For this review, take the finished solid that the model builds, in its own axes (mm). Round coordinates to 2 decimals unless told otherwise and drop trailing zeros. Write each loop counter-clockwise with the first axis right and the second up, starting at its lowest first coordinate (ties: lowest second). Pieces come first, ordered by that corner, then holes. Notation, with made-up numbers: (70.25, 32) - (97.25, 32) arc R21 ccw to (97.25, 66) - close; hole circle Ø4 at (12, 42.5). An arc over 180 degrees is marked (long way). One line per item, written item: value. Start each with the question number.
Q1. Clearance check with flat-ended pins moving along their axes: pin 1 Ø3.5 at (x, y) = (-23.5, -23.5) entering from -Z; pin 2 Ø3.5 at (x, y) = (23.5, 23.5) entering from +Z. State where each tip first meets the part, or that it passes through.
Q2. For probe 1 along Y at (x, z) = (-23.5, 1.4); probe 2 along Y at (x, z) = (22.5, 1.15); probe 3 along X at (y, z) = (23, 1.6), list the stretches that pass through material, from the lowest coordinate up.
Q3. Add section A-A on z = 0.7. Write out the cut boundary in (x, y), and give its area (3 significant figures).
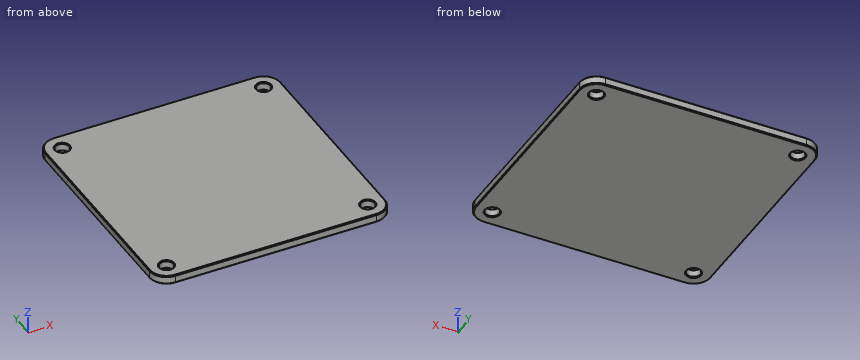
```python
from build123d import *

# Parameters (mm, degrees)
SKETCH3_W           = 55
SKETCH3_H           = 55
BOSS_EXTRUDE1_DEPTH = 2
CUT_EXTRUDE1_DEPTH  = 2
SKETCH6_R           = 1.6
CUT_EXTRUDE2_DEPTH  = 39.942264957
CHAMFER1_SIZE       = 0.2
CHAMFER2_SIZE       = 0.2


with BuildPart() as part:
    # Sketch3 → Boss-Extrude1 (new body)
    with BuildSketch(Plane.XY):
        Rectangle(SKETCH3_W, SKETCH3_H)
    extrude(amount=BOSS_EXTRUDE1_DEPTH)

    # Sketch4 → Cut-Extrude1 (cut)
    with BuildSketch(Plane.XY.offset(2)):
        with BuildLine():
            Line((-23.5, 27.5), (-27.5, 27.5))
            Line((-27.5, 27.5), (-27.5, 23.5))
            ThreePointArc((-27.5, 23.5), (-26.328427125, 26.328427125), (-23.5, 27.5))
        make_face()
        with BuildLine():
            Line((23.5, 27.5), (27.5, 27.5))
            Line((27.5, 27.5), (27.5, 23.5))
            ThreePointArc((27.5, 23.5), (26.328427125, 26.328427125), (23.5, 27.5))
        make_face()
        with BuildLine():
            Line((27.5, -23.5), (27.5, -27.5))
            Line((27.5, -27.5), (23.5, -27.5))
            ThreePointArc((23.5, -27.5), (26.328427125, -26.328427125), (27.5, -23.5))
        make_face()
        with BuildLine():
            Line((-23.5, -27.5), (-27.5, -27.5))
            Line((-27.5, -27.5), (-27.5, -23.5))
            ThreePointArc((-27.5, -23.5), (-26.328427125, -26.328427125), (-23.5, -27.5))
        make_face()
    extrude(amount=-CUT_EXTRUDE1_DEPTH, mode=Mode.SUBTRACT)

    # Sketch6 → Cut-Extrude2 (cut, through all)
    with BuildSketch(Plane.XY.offset(2)):
        with Locations((23.5, 23.5)):
            Circle(SKETCH6_R)
        with Locations(Location((-23.5, 23.5, 0), (0, 0, 180))):
            Circle(SKETCH6_R)
        with Locations(Location((23.5, -23.5, 0), (0, 0, 180))):
            Circle(SKETCH6_R)
        with Locations((-23.5, -23.5)):
            Circle(SKETCH6_R)
    extrude(amount=-CUT_EXTRUDE2_DEPTH, mode=Mode.SUBTRACT)

    # Chamfer1
    chamfer1_edges = [part.edges().sort_by_distance(p)[0] for p in [
        (0, 27.5, 0),
        (26.328427125, 26.328427125, 0),
        (27.5, 0, 0),
        (0, -27.5, 0),
        (-27.5, 0, 0),
        (-26.328427125, 26.328427125, 0),
        (26.328427125, -26.328427125, 0),
        (-26.328427125, -26.328427125, 0),
        (21.9, 23.5, 0),
        (-21.9, 23.5, 0),
        (25.1, -23.5, 0),
        (-25.1, -23.5, 0),
    ]]
    chamfer(chamfer1_edges, length=CHAMFER1_SIZE)

    # Chamfer2
    chamfer2_edges = [part.edges().sort_by_distance(p)[0] for p in [
        (0, 27.5, 2),
        (26.328427125, 26.328427125, 2),
        (-27.5, 0, 2),
        (0, -27.5, 2),
        (27.5, 0, 2),
        (-26.328427125, 26.328427125, 2),
        (26.328427125, -26.328427125, 2),
        (-26.328427125, -26.328427125, 2),
        (21.9, 23.5, 2),
        (-21.9, 23.5, 2),
        (25.1, -23.5, 2),
        (-25.1, -23.5, 2),
    ]]
    chamfer(chamfer2_edges, length=CHAMFER2_SIZE)


solid = part.part
```
Result set:
1. pin 1: stops at z = 0.05
1. pin 2: stops at z = 1.95
2. probe 1: y = -27.5 to -25.1, -21.9 to 21.9, 25.1 to 27.5
2. probe 2: y = -27.5 to -24.75, -22.25 to 22.25, 24.75 to 27.5
2. probe 3: x = -27.5 to -25.02, -21.98 to 21.98, 25.02 to 27.5
3. outline: (-27.5, -23.5) arc R4 ccw to (-23.5, -27.5) - (23.5, -27.5) arc R4 ccw to (27.5, -23.5) - (27.5, 23.5) arc R4 ccw to (23.5, 27.5) - (-23.5, 27.5) arc R4 ccw to (-27.5, 23.5) - close; hole circle Ø3.2 at (-23.5, -23.5); hole circle Ø3.2 at (-23.5, 23.5); hole circle Ø3.2 at (23.5, -23.5); hole circle Ø3.2 at (23.5, 23.5)
3. area: 2,980 mm^2
